Can you work these out from the drawing? Everything is in mm from the part's minimum corner. Coordinates: 2 decimals unless noted, no trailing zeros. Loops run counter-clockwise (first coordinate to the right, second up) from the corner with the lowest first, then second, coordinate; pieces in that order, holes last. Notation, with made-up numbers: (-30, -13) -> (19, -13) arc R24 cw to (19, 21) -> close; hole circle Ø5 at (25, 13). An arc over 180 degrees is marked (long way). Put each result on its own line as item: value. Start each with the question number.
Item 1: If we section it at C-C on z = 54: Please give me the cut outline in (x, y), plus the area to 3 significant figures.
Item 2: If we section it at A-A on x = 85.5: Please give me the cut outline in (y, z).
Item 3: If we section it at B-B on y = 47.5: Please give me the cut outline in (x, z) (1 decimal).
Item 4: Please list where these lines run through material, in increasing order: L1, parallel to Y at x = 75, z = 19.5; L2, parallel to Y at x = 48, z = 11; L3, parallel to Z at x = 83.5, y = 77 (1 decimal). Write a range as from..to.
Item 5: Will these pins go through, and if not, where does the flat tip stop? P1, Ø12, axis at x = 83.5, y = 66.5, coming from the +Z side; P2, Ø1.5, axis at x = 41, z = 20, coming from the +Y side; P3, Ø5, axis at x = 21, y = 77.5, coming from the +Z side (1 decimal).
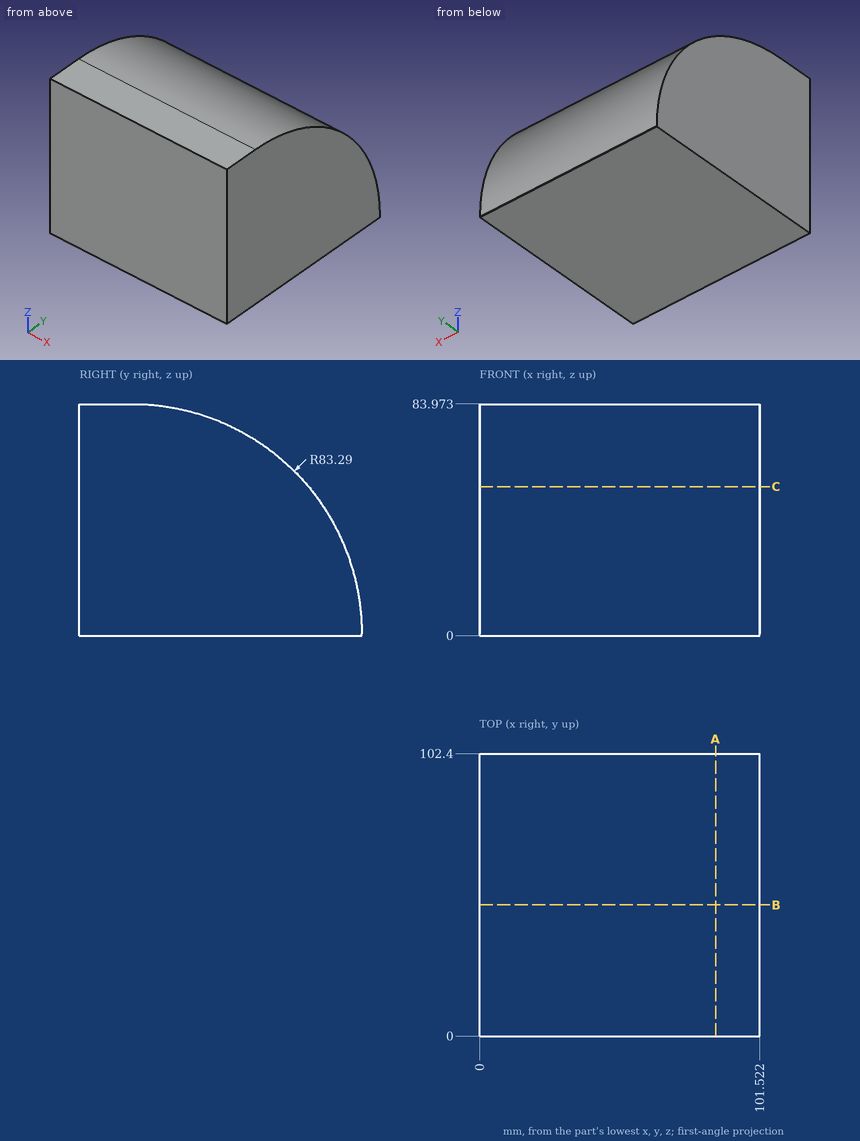
Solutions:
1. outline: (0, 0) -> (101.52, 0) -> (101.52, 83.1) -> (0, 83.1) -> close
1. area: 8,440 mm^2
2. outline: (0, 0) -> (102.4, 0) -> (102.4, 0.68) arc R83.29 ccw to (19.11, 83.97) -> (0, 83.97) -> close
3. outline: (0, 0) -> (101.5, 0) -> (101.5, 79) -> (0, 79) -> close
4. L1: 0..100.25
4. L2: 0..101.76
4. L3: 0..60.6
5. P1: z = 72.96
5. P2: y = 100.3
5. P3: z = 62.4
